Input: part model. Units: mm. Frame: model coordinates. Face numbers are marked on the shaded views. Coordinates: 2 decimals unless noted, no trailing zeros. Loops run counter-clockwise (first coordinate to the right, second up) from the corner with the lowest first, then second, coordinate; pieces in that order, holes last.
Autodesk Inventor part; units mm, degrees
ref_plane "YZ Plane" through (0, 0, 0) normal (1, 0, 0) x (0, 1, 0)
ref_plane "XZ Plane" through (0, 0, 0) normal (0, 1, 0) x (-1, 0, 0)
ref_plane "XY Plane" through (0, 0, 0) normal (0, 0, 1) x (1, 0, 0)
sketch "Sketch1" plane through (0, 0, 0) normal (0, 1, 0) x (-1, 0, 0)
  line L0 (17.75, 24) -> (-17.75, 24)
  line L1 (-17.75, 24) -> (-17.75, -24)
  line L2 (-17.75, -24) -> (17.75, -24)
  line L3 (17.75, -24) -> (17.75, 24)
  line L4 (17.75, 24) -> (-17.75, -24) construction
  line L5 (-17.75, 24) -> (17.75, -24) construction
  point P0 (0, 0)
  dimension "d0" = 35.5
  dimension "d1" = 48
extrude "Extrusion1" add sketch "Sketch1" along normal blind 1.6
sketch "Sketch2" plane through (0, 1.6, 0) normal (0, 1, 0) x (1, 0, 0)
  line L0 (-12, 19.5) -> (-8, 19.5)
  line L1 (-8, 19.5) -> (-8, 15.5)
  line L2 (-8, 15.5) -> (-12, 15.5)
  line L3 (-12, 15.5) -> (-12, 19.5)
  line L4 (-12, 19.5) -> (-8, 15.5) construction
  line L5 (-8, 19.5) -> (-12, 15.5) construction
  line L6 (-17.75, -24) -> (17.75, -24)
  line L7 (17.75, 24) -> (-17.75, 24)
  line L8 (-17.75, 24) -> (-17.75, -24)
  line L9 (17.75, -24) -> (17.75, 24)
  line L10 (12, 15.5) -> (8, 15.5)
  line L11 (12, 19.5) -> (12, 15.5)
  line L12 (8, 19.5) -> (12, 19.5)
  line L13 (8, 15.5) -> (8, 19.5)
  line L14 (-8, 8.5) -> (-12, 8.5)
  line L15 (-8, 12.5) -> (-8, 8.5)
  line L16 (-12, 12.5) -> (-8, 12.5)
  line L17 (-12, 8.5) -> (-12, 12.5)
  line L18 (12, 8.5) -> (8, 8.5)
  line L19 (12, 12.5) -> (12, 8.5)
  line L20 (8, 12.5) -> (12, 12.5)
  line L21 (8, 8.5) -> (8, 12.5)
  line L22 (-8, 1.5) -> (-12, 1.5)
  line L23 (-8, 5.5) -> (-8, 1.5)
  line L24 (-12, 5.5) -> (-8, 5.5)
  line L25 (-12, 1.5) -> (-12, 5.5)
  line L26 (12, 1.5) -> (8, 1.5)
  line L27 (12, 5.5) -> (12, 1.5)
  line L28 (8, 5.5) -> (12, 5.5)
  line L29 (8, 1.5) -> (8, 5.5)
  line L30 (-8, -5.5) -> (-12, -5.5)
  line L31 (-8, -1.5) -> (-8, -5.5)
  line L32 (-12, -1.5) -> (-8, -1.5)
  line L33 (-12, -5.5) -> (-12, -1.5)
  line L34 (12, -5.5) -> (8, -5.5)
  line L35 (12, -1.5) -> (12, -5.5)
  line L36 (8, -1.5) -> (12, -1.5)
  line L37 (8, -5.5) -> (8, -1.5)
  line L38 (-8, -12.5) -> (-12, -12.5)
  line L39 (-8, -8.5) -> (-8, -12.5)
  line L40 (-12, -8.5) -> (-8, -8.5)
  line L41 (-12, -12.5) -> (-12, -8.5)
  line L42 (12, -12.5) -> (8, -12.5)
  line L43 (12, -8.5) -> (12, -12.5)
  line L44 (8, -8.5) -> (12, -8.5)
  line L45 (8, -12.5) -> (8, -8.5)
  line L46 (-8, -19.5) -> (-12, -19.5)
  line L47 (-8, -15.5) -> (-8, -19.5)
  line L48 (-12, -15.5) -> (-8, -15.5)
  line L49 (-12, -19.5) -> (-12, -15.5)
  line L50 (12, -19.5) -> (8, -19.5)
  line L51 (12, -15.5) -> (12, -19.5)
  line L52 (8, -15.5) -> (12, -15.5)
  line L53 (8, -19.5) -> (8, -15.5)
  point P0 (0, 0)
  point P1 (-10, 17.5)
  dimension "d4" = 4
  dimension "d5" = 4
  dimension "d6" = 48
  dimension "d7" = 35.5
  dimension "d8" = 17.5
  dimension "d9" = 10
  dimension "d20" = 20
  dimension "d23" = 7
extrude "Extrusion2" add sketch "Sketch2" along normal blind 1.6 contours L0 L1 L2 L3 | L10 L13 L12 L11 | L14 L17 L16 L15 | L18 L21 L20 L19 | L22 L25 L24 L23 | L26 L29 L28 L27 | L30 L33 L32 L31 | L34 L37 L36 L35 | L38 L41 L40 L39 | L42 L45 L44 L43 | L46 L49 L48 L47 | L50 L53 L52 L51
sketch "Sketch3" plane through (0, 1.6, 0) normal (0, 1, 0) x (1, 0, 0)
  line L0 (0, 0) -> (0, 19.05) construction
  line L1 (0, 0) -> (4.4844, 0) construction
  circle A0 centre (0, 19.05) radius 1.1
  circle A1 centre (0, -19.05) radius 1.1
  dimension "d28" = 19.05
  dimension "d29" = 2.2
extrude "Extrusion3" cut sketch "Sketch3" against normal through all
properties part number "RedLEDArray"
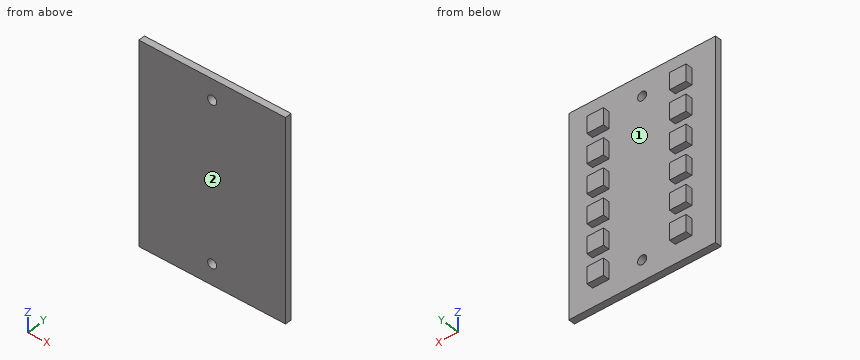
Item 1: Contact query for flat-ended pins moving along their axis: P1, Ø3.5, axis at x = 0, z = 19.05, coming from the +Y side; P2, Ø1, axis at x = 1.5, y = 2.5, coming from the -Z side; P3, Ø0.5, axis at y = 2.5, z = 9.5, coming from the -X side; P4, Ø0.5, axis at x = -10.5, y = 2.5, coming from the +Z side. Output: stop coordinate, or through.
Result:
P1: stops at y = 1.6
P2: passes through
P3: stops at x = -12
P4: stops at z = 19.5
Item 2: Section query D-D (x = -14.5). Output: boundary loops of the cut face in (y, z).
Result:
outline: (0, -24) - (1.6, -24) - (1.6, 24) - (0, 24) - close
Item 3: Section query B-B (y = 2.65). Count the separate pieces of the cut face and the enclosed holes in it, then the cut area to 3 significant figures.
Result:
separate pieces: 12
enclosed holes: 0
area: 192 mm2
Item 4: Mould query, pull axis X, two halves, no side actions, for the marked faces 1 and 2. Classes: +X half, -X half, draft (parallel to the pull), parting line (faces both ways), or undercut.
Result:
face 1: undercut
face 2: draft
Item 5: Line query: L1, parallel to Z at x = 0, y = 0.6; L2, parallel to Z at x = -10.5, y = 2.05; L3, parallel to X at y = 0.9, z = 19.05. Output: solid intervals per line, ascending.
Result:
L1: z = -24 to -20.15, -17.95 to 17.95, 20.15 to 24
L2: z = -19.5 to -15.5, -12.5 to -8.5, -5.5 to -1.5, 1.5 to 5.5, 8.5 to 12.5, 15.5 to 19.5
L3: x = -17.75 to -1.1, 1.1 to 17.75
Item 6: Section query A-A (x = 0). Output: boundary loops of the cut face in (y, z).
Result:
outline: (0, -24) - (1.6, -24) - (1.6, -20.15) - (0, -20.15) - close; (0, -17.95) - (1.6, -17.95) - (1.6, 17.95) - (0, 17.95) - close; (0, 20.15) - (1.6, 20.15) - (1.6, 24) - (0, 24) - close
Item 7: Section query C-C (z = -10.5). Output: boundary loops of the cut face in (x, y), then the cut area to 3 significant figures.
Result:
outline: (-17.75, 0) - (17.75, 0) - (17.75, 1.6) - (12, 1.6) - (12, 3.2) - (8, 3.2) - (8, 1.6) - (-8, 1.6) - (-8, 3.2) - (-12, 3.2) - (-12, 1.6) - (-17.75, 1.6) - close
area: 69.6 mm2
